Part print with two shaded views. Sizes in mm from the minimum x, y, z corner. A direction names the side the tool comes from. Round coordinates to 2 decimals unless told otherwise and drop trailing zeros. Loops run counter-clockwise (first coordinate to the right, second up) from the corner with the lowest first, then second, coordinate; pieces in that order, holes last.
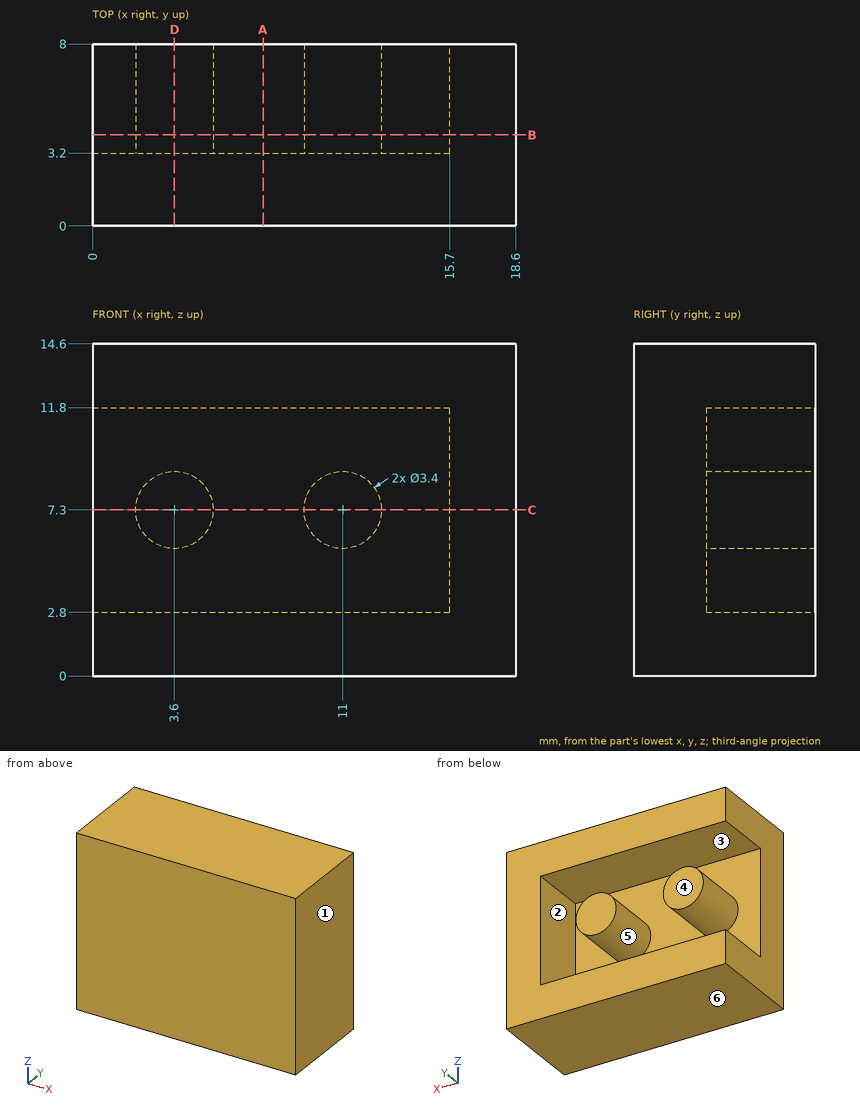
Item 1: Mould opens along Z. For the marked faces 4, 5 and 6 say: released by +Z, released by -Z, zero draft, split by the parting line, or undercut.
Verdict:
face 4: zero draft
face 5: undercut
face 6: released by -Z
Item 2: Cut at D-D (x = 3.6). List the corners of the cut face in (y, z), plus the area to 3 significant figures.
Verdict:
outline: (0, 0) - (8, 0) - (8, 2.8) - (3.2, 2.8) - (3.2, 5.6) - (8, 5.6) - (8, 9) - (3.2, 9) - (3.2, 11.8) - (8, 11.8) - (8, 14.6) - (0, 14.6) - close
area: 89.9 mm2
Item 3: Cut at A-A (x = 7.5). List the corners of the cut face in (y, z), plus the area to 3 significant figures.
Verdict:
outline: (0, 0) - (8, 0) - (8, 2.8) - (3.2, 2.8) - (3.2, 11.8) - (8, 11.8) - (8, 14.6) - (0, 14.6) - close
area: 73.6 mm2
Item 4: Flat gauge pin, fed straight in: P1, Ø4.5, axis at x = 5, z = 9, coming from the +Y side. Where does the tip first touch, or does it go through?
Verdict:
P1: stops at y = 8
Item 5: Cut at C-C (z = 7.3). List the corners of the cut face in (x, y), plus the area to 3 significant figures.
Verdict:
outline: (0, 0) - (18.6, 0) - (18.6, 8) - (15.7, 8) - (15.7, 3.2) - (12.7, 3.2) - (12.7, 8) - (9.3, 8) - (9.3, 3.2) - (5.3, 3.2) - (5.3, 8) - (1.9, 8) - (1.9, 3.2) - (0, 3.2) - close
area: 106 mm2
Item 6: Cut at B-B (y = 4). List the corners of the cut face in (x, z).
Verdict:
outline: (0, 0) - (18.6, 0) - (18.6, 14.6) - (0, 14.6) - (0, 11.8) - (15.7, 11.8) - (15.7, 2.8) - (0, 2.8) - close; circle Ø3.4 at (3.6, 7.3); circle Ø3.4 at (11, 7.3)
Item 7: Wall check: L1, parallel to Z at x = 14, y = 6; L2, parallel to Z at x = 10, y = 3.25; L3, parallel to Z at x = 3, y = 5.75. Give the ranges that are in metal, low to high.
Verdict:
L1: z = 0 to 2.8, 11.8 to 14.6
L2: z = 0 to 2.8, 5.93 to 8.67, 11.8 to 14.6
L3: z = 0 to 2.8, 5.71 to 8.89, 11.8 to 14.6
Item 8: 3-axis set-ups, long thin cutter, end or side, ignore diameter. For the marked faces 1, 2 and 3: which of +Z, -Z, +X, -X, +Y, -Y reach the whole face in a straight line?
Verdict:
face 1: +Z, -Z, +X, +Y, -Y
face 2: +Y
face 3: -X, +Y
